from build123d import *

# Parameters (mm, degrees)
F0_W     = 49
F0_H     = 33.5
F0_R     = 3.75
F1_DEPTH = 9.5
F2_R     = 7
F4_R     = 3
F3_W     = 49
F3_H     = 3.5
F5_DEPTH = 14
F7_DEPTH = 50


with BuildPart() as f1:
    # F0 (on Top) → F1 (new body)
    with BuildSketch(Plane.XY):
        with Locations((3.22683, 3.281258)):
            Rectangle(F0_W, F0_H)
        with Locations((-10.52317, -2.718742)):
            Circle(F0_R, mode=Mode.SUBTRACT)
        with Locations((16.97683, -2.718742)):
            Circle(F0_R, mode=Mode.SUBTRACT)
    extrude(amount=F1_DEPTH)

    # F2
    f2_edges = [f1.edges().sort_by_distance(p)[0] for p in [
        (-21.27317, -13.468742, 4.75),
        (27.72683, -13.468742, 4.75),
    ]]
    fillet(f2_edges, radius=F2_R)

    # F4
    f4_edges = [f1.edges().sort_by_distance(p)[0] for p in [
        (27.72683, 20.031258, 4.75),
        (-21.27317, 20.031258, 4.75),
    ]]
    fillet(f4_edges, radius=F4_R)

    # F3 (on face) → F5 (cut)
    with BuildSketch(Plane(origin=(0, 20.031258, 0), x_dir=(-1, 0, 0), z_dir=(0, 1, 0))):
        with Locations((-3.22683, 4.75)):
            Rectangle(F3_W, F3_H)
    extrude(amount=-F5_DEPTH, mode=Mode.SUBTRACT)

    # F6 (on face) → F7 (cut)
    with BuildSketch(Plane.YZ.offset(27.72683)):
        with BuildLine():
            ThreePointArc((7.577891, 6.5), (6.804574, 7.273316), (6.031258, 6.5))
            Line((6.031258, 6.5), (7.577891, 6.5))
        make_face()
        with BuildLine():
            Line((7.577891, 3), (6.031258, 3))
            ThreePointArc((6.031258, 3), (6.804574, 2.226684), (7.577891, 3))
        make_face()
    extrude(amount=-F7_DEPTH, mode=Mode.SUBTRACT)


solid = f1.part
Here's how the part is built. I have some questions about the finished solid (model axes, mm). A direction names the side the tool comes from. Round coordinates to 2 decimals unless told otherwise and drop trailing zeros. Order: outer loops, then holes, each group sorted by start corner. A loop starts at its lowest first (then second) coordinate and runs counter-clockwise, first axis right, second up. Notation, with made-up numbers: (64.5, -39.5) -> (97.5, -39.5) arc R7 ccw to (97.5, -31.5) -> close; hole circle Ø7 at (22, 36.5). An arc over 180 degrees is marked (long way). Use CSV: the item, a comma, the result in double quotes.
1. I want a section at D-D on z = 6. List the corners of the cut face in (x, y) for me.
Recorded:
outline,"(-21.27, -6.47) arc R7 ccw to (-14.27, -13.47) -> (20.73, -13.47) arc R7 ccw to (27.73, -6.47) -> (27.73, 6.03) -> (-21.27, 6.03) -> close; hole circle Ø7.5 at (-10.52, -2.72); hole circle Ø7.5 at (16.98, -2.72)"
2. I want a section at C-C on x = 4. List the corners of the cut face in (y, z) for me.
Recorded:
outline,"(-13.47, 0) -> (20.03, 0) -> (20.03, 3) -> (7.58, 3) arc R0.77 cw to (6.03, 3) -> (6.03, 6.5) arc R0.77 cw to (7.58, 6.5) -> (20.03, 6.5) -> (20.03, 9.5) -> (-13.47, 9.5) -> close"
3. Thinking about a two-plate mould opening in Z: for faces 4 (the face through (4, 14, 3)), 5 (the face through (4, 14, 6.5)), 6 (the face through (3, 4, 0)), 7 (the face through (-20.418, 19.129, 8.021)), which applies, pulls with the +Z half, pulls with the -Z half, needs draft (parallel to the pull), parting line crosses it, or undercut?
Recorded:
face 4,"undercut"
face 5,"undercut"
face 6,"pulls with the -Z half"
face 7,"needs draft"
4. I want a section at B-B on z = 1.25. List the corners of the cut face in (x, y) for me.
Recorded:
outline,"(-21.27, -6.47) arc R7 ccw to (-14.27, -13.47) -> (20.73, -13.47) arc R7 ccw to (27.73, -6.47) -> (27.73, 17.03) arc R3 ccw to (24.73, 20.03) -> (-18.27, 20.03) arc R3 ccw to (-21.27, 17.03) -> close; hole circle Ø7.5 at (-10.52, -2.72); hole circle Ø7.5 at (16.98, -2.72)"
5. Which directions (+Z, -Z, +X, -X, +Y, -Y) give clear straight access to the entire face, cutting with the end or side of a thin tool? Please do faces 1 (the face through (3.57, 6.822, 7.273)), 2 (the face through (26.8, 19.2, 1.5)), 3 (the face through (4, 6.031, 5)).
Recorded:
face 1,"+X, -X"
face 2,"+Z, -Z, +X, +Y"
face 3,"+X, -X, +Y"
6. I need wall thicknesses on line 1 along X through (y, z) = (-2.5, 3.25); line 2 along Z through (x, y) = (11.5, 9.5); line 3 along X through (y, z) = (-4, 8). Which ranges of each line are inside material? Lowest first, please.
Recorded:
line 1,"x = -21.27 to -14.27, -6.78 to 13.23, 20.72 to 27.73"
line 2,"z = 0 to 3, 6.5 to 9.5"
line 3,"x = -21.27 to -14.05, -7 to 13.45, 20.5 to 27.73"
7. I want a section at A-A on x = -13. List the corners of the cut face in (y, z) for me.
Recorded:
outline,"(-13.47, 0) -> (-5.53, 0) -> (-5.53, 9.5) -> (-13.47, 9.5) -> close; (0.1, 0) -> (20.03, 0) -> (20.03, 3) -> (7.58, 3) arc R0.77 cw to (6.03, 3) -> (6.03, 6.5) arc R0.77 cw to (7.58, 6.5) -> (20.03, 6.5) -> (20.03, 9.5) -> (0.1, 9.5) -> close"
